Autodesk Inventor part; units mm, degrees
ref_plane "YZ Plane" through (0, 0, 0) normal (1, 0, 0) x (0, 1, 0)
ref_plane "XZ Plane" through (0, 0, 0) normal (0, 1, 0) x (-1, 0, 0)
ref_plane "XY Plane" through (0, 0, 0) normal (0, 0, 1) x (1, 0, 0)
sketch "Sketch1" plane through (0, 0, 0) normal (0, 0, 1) x (1, 0, 0)
  circle A0 centre (0, 0) radius 40
  circle A1 centre (0, 0) radius 27
  circle A2 centre (0, 0) radius 17
  circle A3 centre (0, 33) radius 3.3
  circle A4 centre (-33, 0) radius 3.3
  circle A5 centre (0, -33) radius 3.3
  circle A6 centre (33, 0) radius 3.3
  dimension "d0" = 80
  dimension "d1" = 54
  dimension "d2" = 34
  dimension "d4" = 6.6
  dimension "d5" = 6.6
  dimension "d6" = 6.6
  dimension "d7" = 6.6
extrude "Extrusion1" add sketch "Sketch1" along normal blind 2 contours A0
extrude "Extrusion2" add sketch "Sketch1" along normal blind 8 contours A1
properties part number "tensorpolea"
Geometry check sheet. Reference: the model listing, model coordinates, mm. A direction names the side the tool comes from. Coordinates: 2 decimals unless noted, no trailing zeros. Order: outer loops, then holes, each group sorted by start corner. A loop starts at its lowest first (then second) coordinate and runs counter-clockwise, first axis right, second up.
Item 1: Section check B-B (x = 31.5). Enter the section's corners in (y, z).
Item 2: Section check D-D (y = -33). Enter the section's corners in (x, z).
Item 3: Section check A-A (x = 0). Enter the section's corners in (y, z).
Item 4: Tool access check on faces 4 (the flat face through (26, -8, 2)), 5 (the cylindrical face through (-8.67, 39.05, 0.99)). Record the directions out of +Z, -Z, +X, -X, +Y, -Y that give a thin tool (end or side, any length) a straight path to the whole face; none if there is none.
Item 5: Mould release check, pull along Y, two halves, no side actions. Record for faces 1 (the cylindrical face through (-0.72, 36.22, 0.99)), 2 (the cylindrical face through (-5.85, 26.36, 4.96)), 3 (the flat face through (18, 0, 8)): released by +Y, released by -Y, zero draft, split by the parting line, or undercut.
Item 6: Section check C-C (z = 1). Enter the section's corners in (x, y).
Item 7: Depth check by flat-ended pin: pin 1 (1.5 mm diameter, centred on x = -7, z = 7, fed in from +Y); pin 2 (1.5 mm diameter, centred on x = -15.5, z = 6, fed in from -Y) (3 decimals); pin 3 (4 mm diameter, centred on y = -12.5, z = 3, fed in from +X); pin 4 (4 mm diameter, centred on x = -33, y = 0, fed in from -Z). Enter the tip coordinate at first touch or a pass-through.
Item 8: Scan lines: line 1 along Y through (x, z) = (0, 4.25); line 2 along Z through (x, y) = (-3, -31); line 3 along Y through (x, z) = (-8.5, 6). Record each from-to range of solid material in increasing order.
Check sheet entries:
1. outline: (-24.65, 0) - (-2.94, 0) - (-2.94, 2) - (-24.65, 2) - close; (2.94, 0) - (24.65, 0) - (24.65, 2) - (2.94, 2) - close
2. outline: (-22.61, 0) - (-3.3, 0) - (-3.3, 2) - (-22.61, 2) - close; (3.3, 0) - (22.61, 0) - (22.61, 2) - (3.3, 2) - close
3. outline: (-40, 0) - (-36.3, 0) - (-36.3, 2) - (-40, 2) - close; (-29.7, 0) - (-17, 0) - (-17, 8) - (-27, 8) - (-27, 2) - (-29.7, 2) - close; (17, 0) - (29.7, 0) - (29.7, 2) - (27, 2) - (27, 8) - (17, 8) - close; (36.3, 0) - (40, 0) - (40, 2) - (36.3, 2) - close
4. face 4: +Z
4. face 5: +Z, -Z
5. face 1: undercut
5. face 2: split by the parting line
5. face 3: zero draft
6. outline: circle Ø80 at (0, 0); hole circle Ø6.6 at (-33, 0); hole circle Ø34 at (0, 0); hole circle Ø6.6 at (0, -33); hole circle Ø6.6 at (0, 33); hole circle Ø6.6 at (33, 0)
7. pin 1: stops at y = 26.27
7. pin 2: stops at y = -22.615
7. pin 3: stops at x = 38.52
7. pin 4: passes through
8. line 1: y = -27 to -17, 17 to 27
8. line 2: z = 0 to 2
8. line 3: y = -25.63 to -14.72, 14.72 to 25.63
